Verification items for this drawing (mm, ordinates from the low corner). A direction names the side the tool comes from. Round coordinates to 2 decimals unless told otherwise and drop trailing zeros. Order: outer loops, then holes, each group sorted by start corner. A loop starts at its lowest first (then second) coordinate and runs counter-clockwise, first axis right, second up. Notation, with made-up numbers: (75, 35) -> (111, 35) arc R8 ccw to (111, 43) -> close; hole circle Ø11 at (-7.75, 5). An arc over 180 degrees is marked (long way). Answer in a Markdown table with one row per item. Add a question column.
1. Sectioned sample at A-A, the plane y = 33. Record the boundary of the cut face in (x, z), then the cut area to 3 significant figures.
2. Material ranges on L1, parallel to X at y = 16, z = 2.1; L2, parallel to Y at x = 4.25, z = 1.3 (1 decimal); L3, parallel to Y at x = 5.25, z = 1.1 (1 decimal), recorded low to high. Write a range as from..to.
3. Sectioned sample at B-B, the plane z = 1.2. Record the boundary of the cut face in (x, y), then the cut area to 3 significant figures.
4. Access from +Z, -Z, +X, -X, +Y, -Y to the whole of each face (thin tool, end or side, straight path). Record for the marked faces 1 and 2.
5. Sectioned sample at C-C, the plane y = 24. Record the boundary of the cut face in (x, z), then the cut area to 3 significant figures.
6. Depth check by flat-ended pin: P1, Ø4, axis at x = 5, y = 33, coming from the +Z side; P2, Ø1.5, axis at y = 8.5, z = 1.5, coming from the -X side. Enter the tip coordinate at first touch or a pass-through.
7. Draft check along Y on the marked faces 3, 4 and 5. Enter one of: +Y half, -Y half, draft (parallel to the pull), parting line (faces both ways), or undercut.
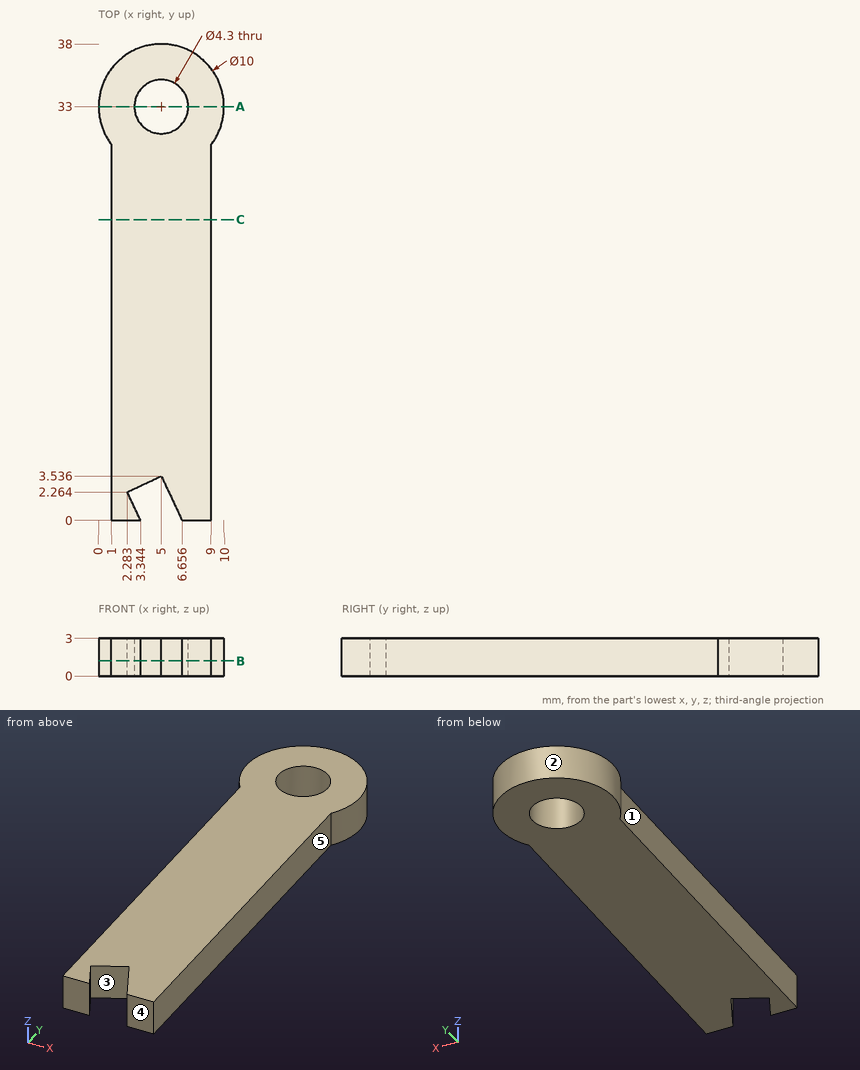
Answer key:
| question | item | result |
|---|---|---|
| 1 | outline | (0, 0) -> (2.85, 0) -> (2.85, 3) -> (0, 3) -> close; (7.15, 0) -> (10, 0) -> (10, 3) -> (7.15, 3) -> close |
| 1 | area | 17.1 mm² |
| 2 | L1 | x = 1..9 |
| 2 | L2 | y = 3.2..31, 35..37.9 |
| 2 | L3 | y = 3..30.9, 35.1..38 |
| 3 | outline | (1, 0) -> (3.34, 0) -> (2.28, 2.26) -> (5, 3.54) -> (6.66, 0) -> (9, 0) -> (9, 30) arc R5 ccw (long way) to (1, 30) -> close; hole circle Ø4.3 at (5, 33) |
| 3 | area | 283 mm² |
| 4 | face 1 | +Z, -Z, -X, -Y |
| 4 | face 2 | +Z, -Z |
| 5 | outline | (1, 0) -> (9, 0) -> (9, 3) -> (1, 3) -> close |
| 5 | area | 24.0 mm² |
| 6 | P1 | passes through |
| 6 | P2 | stops at x = 1 |
| 7 | face 3 | undercut |
| 7 | face 4 | -Y half |
| 7 | face 5 | draft |
